Autodesk Inventor part; units mm, degrees
ref_plane "YZ Plane" through (0, 0, 0) normal (1, 0, 0) x (0, 1, 0)
ref_plane "XZ Plane" through (0, 0, 0) normal (0, 1, 0) x (-1, 0, 0)
ref_plane "XY Plane" through (0, 0, 0) normal (0, 0, 1) x (1, 0, 0)
sketch "Sketch1" plane through (0, 0, 0) normal (0, 0, 1) x (1, 0, 0)
  line L0 (-609.6, 914.4) -> (609.6, 914.4)
  line L1 (609.6, 914.4) -> (609.6, 0)
  line L2 (609.6, 0) -> (-609.6, 0)
  line L3 (-609.6, 0) -> (-609.6, 914.4)
  point P0 (0, 0)
  dimension "d0" = 1219.2
  dimension "d1" = 914.4
  dimension "d2" = 914.4
  dimension "d3" = 609.6
extrude "Plywood" add sketch "Sketch1" along normal blind 19.05
sketch "Sketch2" plane through (0, 0, 19.05) normal (0, 0, 1) x (1, 0, 0)
  line L0 (-177.8, 76.2) -> (177.8, 76.2)
  line L1 (177.8, 76.2) -> (177.8, 0)
  line L2 (177.8, 0) -> (-177.8, 0)
  line L3 (-177.8, 0) -> (-177.8, 76.2)
  line L4 (-609.6, 0) -> (609.6, 0)
  line L5 (-381, 558.8) -> (76.2, 558.8)
  line L6 (76.2, 558.8) -> (76.2, 457.2)
  line L7 (76.2, 457.2) -> (-381, 457.2)
  line L8 (-381, 457.2) -> (-381, 558.8)
  line L9 (-381, 508) -> (76.2, 508) construction
  line L10 (279.4, 736.6) -> (381, 736.6)
  line L11 (381, 736.6) -> (381, 279.4)
  line L12 (381, 279.4) -> (279.4, 279.4)
  line L13 (279.4, 279.4) -> (279.4, 736.6)
  line L14 (76.2, 508) -> (279.4, 508)
  point P0 (0, 0)
  dimension "d6" = 355.6
  dimension "d7" = 76.2
  dimension "d8" = 177.8
  dimension "d9" = 457.2
  dimension "d10" = 381
  dimension "d11" = 101.6
  dimension "d12" = 508
  dimension "d15" = 101.6
  dimension "d16" = 457.2
  dimension "d17" = 203.2
  dimension "d18" = 762
extrude "SLOTS" cut sketch "Sketch2" against normal through all
equation "\"d15\" = d11"
equation "\"d16\" = d9"
properties part number "Plywood"
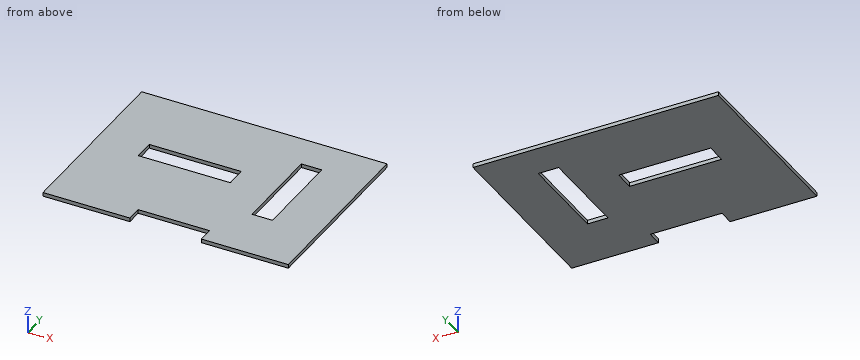
Geometry check sheet. Reference: the model listing, model coordinates, mm. Give positions to 0.01 mm unless a question says otherwise; leave off trailing zeros. Order: outer loops, then holes, each group sorted by start corner. A loop starts at its lowest first (then second) coordinate and runs counter-clockwise, first axis right, second up. Notation, with made-up numbers: M 54,83 L 83,83 A21 cw 83,109 Z; hole C 87.5,-33.5 d9. An arc over 180 degrees is marked long. Use a Markdown table: item, result.
Item 1: Depth check by flat-ended pin: P1, Ø1, axis at x = -264.5, y = 243, coming from the -Z side; P2, Ø9.5, axis at x = -54, z = 9.5, coming from the -Y side. Enter the tip coordinate at first touch or a pass-through.
Answers follow:
| item | result |
|---|---|
| P1 | stops at z = 0 |
| P2 | stops at y = 76.2 |
Item 2: Section check A-A (x = -86.5). Record the cut outline in (y, z), and give its area (3 significant figures).
Answers follow:
| item | result |
|---|---|
| outline | M 76.2,0 L 457.2,0 L 457.2,19.05 L 76.2,19.05 Z; M 558.8,0 L 914.4,0 L 914.4,19.05 L 558.8,19.05 Z |
| area | 14,000 mm2 |
Item 3: Section check B-B (y = 376.5). Record the cut outline in (x, z), and give its area (3 significant figures).
Answers follow:
| item | result |
|---|---|
| outline | M -609.6,0 L 279.4,0 L 279.4,19.05 L -609.6,19.05 Z; M 381,0 L 609.6,0 L 609.6,19.05 L 381,19.05 Z |
| area | 21,300 mm2 |
Item 4: Section check C-C (z = 15). Record the cut outline in (x, y), and give its area (3 significant figures).
Answers follow:
| item | result |
|---|---|
| outline | M -609.6,0 L -177.8,0 L -177.8,76.2 L 177.8,76.2 L 177.8,0 L 609.6,0 L 609.6,914.4 L -609.6,914.4 Z; hole M -381,457.2 L 76.2,457.2 L 76.2,558.8 L -381,558.8 Z; hole M 279.4,279.4 L 381,279.4 L 381,736.6 L 279.4,736.6 Z |
| area | 995,000 mm2 |
Item 5: Section check D-D (x = 109). Record the cut outline in (y, z), and give its area (3 significant figures).
Answers follow:
| item | result |
|---|---|
| outline | M 76.2,0 L 914.4,0 L 914.4,19.05 L 76.2,19.05 Z |
| area | 16,000 mm2 |
Item 6: Material ranges on line 1 along Y through (x, z) = (-334, 11.75); line 2 along X through (y, z) = (542, 4); line 3 along X through (y, z) = (387, 3), recorded low to high.
Answers follow:
| item | result |
|---|---|
| line 1 | y = 0 to 457.2, 558.8 to 914.4 |
| line 2 | x = -609.6 to -381, 76.2 to 279.4, 381 to 609.6 |
| line 3 | x = -609.6 to 279.4, 381 to 609.6 |
